from build123d import *

# Parameters (mm, degrees)
SKETCH1_R           = 6.5
BOSS_EXTRUDE1_DEPTH = 13
BOSS_EXTRUDE2_START = 19.9
SKETCH2_W           = 30
SKETCH2_H           = 37
SKETCH2_R           = 8
BOSS_EXTRUDE2_DEPTH = 13


with BuildPart() as part:
    # Sketch1 → Boss-Extrude1 (new body)
    with BuildSketch(Plane(origin=(0, 0, 0), x_dir=(1, 0, 0), z_dir=(0, 1, 0))):
        with BuildLine():
            Line((-10.098039216, -5.637254902), (19.901960784, -5.637254902))
            Line((19.901960784, -5.637254902), (19.901960784, 29.362745098))
            ThreePointArc((19.901960784, 29.362745098), (4.901960784, 44.362745098), (-10.098039216, 29.362745098))
            Line((-10.098039216, 29.362745098), (-10.098039216, -5.637254902))
        make_face()
        with Locations((4.901960784, 29.362745098)):
            Circle(SKETCH1_R, mode=Mode.SUBTRACT)
    extrude(amount=BOSS_EXTRUDE1_DEPTH)

    # Sketch2 → Boss-Extrude2 (add)
    with BuildSketch(Plane(origin=(0, 0, 0), x_dir=(0, 0, -1), z_dir=(1, 0, 0)).offset(BOSS_EXTRUDE2_START)):
        with Locations((9.362745098, 18.5)):
            Rectangle(SKETCH2_W, SKETCH2_H)
        with Locations((9.362745098, 25)):
            Circle(SKETCH2_R, mode=Mode.SUBTRACT)
    extrude(amount=BOSS_EXTRUDE2_DEPTH)


solid = part.part
Design review of the part built by this model. Coordinates are the model's own, in mm. A direction names the side the tool comes from. Give positions to 0.01 mm unless a question says otherwise; leave off trailing zeros. Loops run counter-clockwise (first coordinate to the right, second up) from the corner with the lowest first, then second, coordinate; pieces in that order, holes last. Notation, with made-up numbers: (33, 70) - (61, 70) arc R26 ccw to (61, 93) - close; hole circle Ø5 at (65, 72.5). An arc over 180 degrees is marked (long way). Write item = value, one per line.
1) Take a section at D-D on y = 35.5. State the section outline as (x, z) points, and give its area (3 significant figures).
Result sheet:
outline = (19.9, -24.36) - (32.9, -24.36) - (32.9, 5.64) - (19.9, 5.64) - close
area = 390 mm2
2) To check wall thickness, follow line 1 (Z direction, x = 25, y = 16); line 2 (X direction, y = 34, z = 2); line 3 (Y direction, x = 11.5, z = -33.5). State the ranges of each line that lie inside material, in increasing order.
Result sheet:
line_1 = -24.36 to 5.64
line_2 = 19.9 to 32.9
line_3 = 0 to 13
3) Take a section at A-A on y = 25. State the section outline as (x, z) points.
Result sheet:
outline = (19.9, -24.36) - (32.9, -24.36) - (32.9, -17.36) - (19.9, -17.36) - close; (19.9, -1.36) - (32.9, -1.36) - (32.9, 5.64) - (19.9, 5.64) - close
4) Take a section at B-B on x = 25. State the section outline as (y, z) points, and give its area (3 significant figures).
Result sheet:
outline = (0, -24.36) - (37, -24.36) - (37, 5.64) - (0, 5.64) - close; hole circle Ø16 at (25, -9.36)
area = 909 mm2
5) Draft analysis for pull direction X (two halves, no side actions). For faces 4 (the face through (7.901, 6.409, -23.596)), 5 (the face through (-10.098, 6, -12)), 6 (the face through (11, 0, -14)), state which applies: +X half, -X half, draft (parallel to the pull), parting line (faces both ways), or undercut.
Result sheet:
face_4 = undercut
face_5 = -X half
face_6 = draft
6) Clearance check with flat-ended pins moving along their axes: pin 1 Ø14.5 at (y, z) = (25, -9.36) entering from -X; pin 2 Ø1 at (x, z) = (4.5, -15) entering from +Y; pin 3 Ø10 at (x, z) = (-1.5, 0.5) entering from -Y; pin 4 Ø10.5 at (x, y) = (25, 26.5) entering from -Z. State where each tip first meets the part, or that it passes through.
Result sheet:
pin_1 = through
pin_2 = 13
pin_3 = 0
pin_4 = -24.36
7) Take a section at C-C on z = -15. State the section outline as (x, y) points, and give its area (3 significant figures).
Result sheet:
outline = (-10.1, 0) - (32.9, 0) - (32.9, 19.32) - (19.9, 19.32) - (19.9, 13) - (-10.1, 13) - close; (19.9, 30.68) - (32.9, 30.68) - (32.9, 37) - (19.9, 37) - close
area = 723 mm2
8) Tool access review of faces 1 (the face through (32.9, 15, -9)), 2 (the face through (19.9, 33.2, -9.2)), 3 (the face through (19.902, 6, -27)): name each direction out of +Z, -Z, +X, -X, +Y, -Y from which nothing blocks a thin tool from reaching the whole face with its end or side.
Result sheet:
face_1 = +Z, -Z, +X, +Y, -Y
face_2 = +Z, -Z, -X, +Y
face_3 = -Z, +X, +Y, -Y
